The model under review builds one solid part; all positions refer to its coordinate system, in mm. Round coordinates to 2 decimals unless told otherwise and drop trailing zeros. Write each loop counter-clockwise with the first axis right and the second up, starting at its lowest first coordinate (ties: lowest second). Pieces come first, ordered by that corner, then holes. Notation, with made-up numbers: (-35.5, 28.25) -> (-7.5, 28.25) arc R16 cw to (-7.5, 40.25) -> close; hole circle Ø7 at (-3, 37). An arc over 180 degrees is marked (long way). Answer in a Markdown table with one row per item. Add a question column.
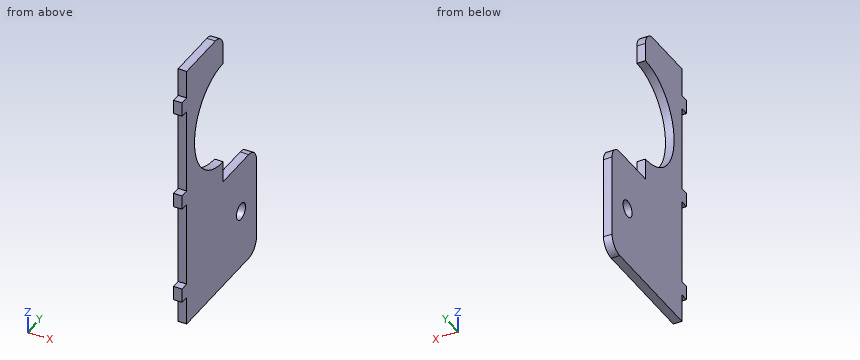
```python
from build123d import *

# Parameters (mm, degrees)
BOSS_EXTRUDE1_DEPTH = 3
SKETCH3_W           = 3
SKETCH3_H           = 5
BOSS_EXTRUDE2_DEPTH = 3
SKETCH5_W           = 3
SKETCH5_H           = 39
BOSS_EXTRUDE3_DEPTH = 21.5
CUT_EXTRUDE3_DEPTH  = 4
FILLET1_R           = 5


with BuildPart() as part:
    # Sketch1 → Boss-Extrude1 (new body)
    with BuildSketch(Plane(origin=(0, 0, 0), x_dir=(0, 0, -1), z_dir=(1, 0, 0))):
        with BuildLine():
            Line((-36, 11.75), (-47.5, 11.75))
            Line((-47.5, 11.75), (-47.5, -11.75))
            Line((-47.5, -11.75), (47.5, -11.75))
            Line((47.5, -11.75), (47.5, 11.75))
            Line((47.5, 11.75), (1, 11.75))
            ThreePointArc((1, 11.75), (-17.5, -6.75), (-36, 11.75))
        make_face()
    extrude(amount=BOSS_EXTRUDE1_DEPTH)

    # Sketch3 → Boss-Extrude2 (add)
    with BuildSketch(Plane.XZ.offset(11.75)):
        with Locations((1.5, -35)):
            Rectangle(SKETCH3_W, SKETCH3_H)
        with Locations((1.5, 0)):
            Rectangle(SKETCH3_W, SKETCH3_H)
        with Locations((1.5, 35)):
            Rectangle(SKETCH3_W, SKETCH3_H)
    extrude(amount=BOSS_EXTRUDE2_DEPTH)

    # Sketch5 → Boss-Extrude3 (add)
    with BuildSketch(Plane(origin=(0, 11.75, 0), x_dir=(1, 0, 0), z_dir=(0, 1, 0))):
        with Locations((1.5, 28)):
            Rectangle(SKETCH5_W, SKETCH5_H)
    extrude(amount=BOSS_EXTRUDE3_DEPTH)

    # Sketch7 → Cut-Extrude3 (cut, through all)
    with BuildSketch(Plane.ZY):
        with BuildLine():
            ThreePointArc((-29.7, 23.25), (-26.8, 20.35), (-23.9, 23.25))
            ThreePointArc((-23.9, 23.25), (-26.8, 26.15), (-29.7, 23.25))
        make_face()
    extrude(amount=-CUT_EXTRUDE3_DEPTH, mode=Mode.SUBTRACT)

    # Fillet1
    fillet1_edges = [part.edges().sort_by_distance(p)[0] for p in [
        (1.5, 11.75, 47.5),
        (1.5, 33.25, -47.5),
        (1.5, 33.25, -8.5),
    ]]
    fillet(fillet1_edges, radius=FILLET1_R)


solid = part.part
```
1. Add section D-D on z = 17.5. Write out the cut boundary in (x, y), plus the area to 3 significant figures.
2. For L1, parallel to Y at x = 1.35, z = -26.8; L2, parallel to Z at x = 2.6, y = 18.5; L3, parallel to Z at x = 2.55, y = 21, list the stretches that pass through material, from the lowest coordinate up.
3. Add section B-B on x = 2.15. Write out the cut boundary in (y, z), plus the area to 3 significant figures.
4. Insertion check: pin 1 Ø1.5 at (x, z) = (1, -4.5) entering from +Y; pin 2 Ø0.9 at (x, z) = (1, 13) entering from -Y; pin 3 Ø0.9 at (x, y) = (2, 20.5) entering from +Z; pin 4 Ø9.5 at (y, z) = (23.25, -26.8) entering from -X. Each pin has a flat end and moves straight along its axis. Give the tip position at first contact, or say it passes through.
5. Add section A-A on z = -26.8. Write out the cut boundary in (x, y).
6. Add section C-C on y = 23.25. Write out the cut boundary in (x, z), plus the area to 3 significant figures.
Filled in:
| question | item | result |
|---|---|---|
| 1 | outline | (0, -11.75) -> (3, -11.75) -> (3, -6.75) -> (0, -6.75) -> close |
| 1 | area | 15.0 mm² |
| 2 | L1 | -11.75 to 20.35, 26.15 to 33.25 |
| 2 | L2 | -47.5 to -8.5 |
| 2 | L3 | -47.5 to -28.63, -24.97 to -8.5 |
| 3 | outline | (-14.75, -37.5) -> (-11.75, -37.5) -> (-11.75, -47.5) -> (28.25, -47.5) arc R5 ccw to (33.25, -42.5) -> (33.25, -13.5) arc R5 ccw to (28.25, -8.5) -> (11.75, -8.5) -> (11.75, -1) arc R18.5 cw to (11.75, 36) -> (11.75, 42.5) arc R5 ccw to (6.75, 47.5) -> (-11.75, 47.5) -> (-11.75, 37.5) -> (-14.75, 37.5) -> (-14.75, 32.5) -> (-11.75, 32.5) -> (-11.75, 2.5) -> (-14.75, 2.5) -> (-14.75, -2.5) -> (-11.75, -2.5) -> (-11.75, -32.5) -> (-14.75, -32.5) -> close; hole circle Ø5.8 at (23.25, -26.8) |
| 3 | area | 2,540 mm² |
| 4 | pin 1 | y = 11.75 |
| 4 | pin 2 | y = -11.75 |
| 4 | pin 3 | z = -8.5 |
| 4 | pin 4 | x = 0 |
| 5 | outline | (0, -11.75) -> (3, -11.75) -> (3, 20.35) -> (0, 20.35) -> close; (0, 26.15) -> (3, 26.15) -> (3, 33.25) -> (0, 33.25) -> close |
| 6 | outline | (0, -47.5) -> (3, -47.5) -> (3, -29.7) -> (0, -29.7) -> close; (0, -23.9) -> (3, -23.9) -> (3, -8.5) -> (0, -8.5) -> close |
| 6 | area | 99.6 mm² |
